from build123d import *

# Parameters (mm, degrees)
DODANIE_WYCI_GNI_CIE1_DEPTH      = 345
DODANIE_WYCI_GNI_CIE1_DEPTH_BACK = 345
SZKIC1_W                         = 200
SZKIC1_H                         = 600
SZKIC2_R                         = 6
SZKIC2_W                         = 660
SZKIC2_H                         = 300
WYTNIJ_WYCI_GNI_CIE1_DEPTH       = 500.024047517
WYTNIJ_WYCI_GNI_CIE2_DEPTH       = 760.012516366
WYTNIJ_WYCI_GNI_CIE3_DEPTH       = 760.012516366
SZKIC5_W                         = 660
SZKIC5_H                         = 130
WYTNIJ_WYCI_GNI_CIE5_DEPTH       = 469.001068375
ZAOKR_GLENIE1_R                  = 20
LUSTRO1_START                    = 330
LUSTRO1_DEPTH                    = 15
LUSTRO1_2_DEPTH                  = 15


# Read off the part's stored shape, not the designer's step: Lustro1
with BuildPart() as part:
    # Szkic1 → Dodanie-wyciągnięcie1 (new, two sides: drawn at the far end of the back side and taken through both)
    with BuildSketch(Plane(origin=(0, 0, 0), x_dir=(0, 0, -1), z_dir=(1, 0, 0)).offset(-DODANIE_WYCI_GNI_CIE1_DEPTH_BACK)):
        Rectangle(SZKIC1_W, SZKIC1_H)
    extrude(amount=DODANIE_WYCI_GNI_CIE1_DEPTH + DODANIE_WYCI_GNI_CIE1_DEPTH_BACK)

    # Szkic2 → Wytnij-wyciągnięcie1 (cut, through all)
    with BuildSketch(Plane.XY.offset(100)):
        with Locations((-150, 240)):
            Circle(SZKIC2_R)
        with Locations((-150, 60)):
            Circle(SZKIC2_R)
        with Locations((150, 60)):
            Circle(SZKIC2_R)
        with Locations((150, 240)):
            Circle(SZKIC2_R)
        with Locations((0, -150)):
            Rectangle(SZKIC2_W, SZKIC2_H)
    extrude(amount=-WYTNIJ_WYCI_GNI_CIE1_DEPTH, mode=Mode.SUBTRACT)

    # Szkic3 → Wytnij-wyciągnięcie2 (cut, through all)
    with BuildSketch(Plane.ZY.offset(345)):
        Polygon((45, -110), (100, -165), (100, 300), (45, 300), align=None)
        Polygon((30, 300), (-100, 0), (-100, 300), align=None)
    extrude(amount=-WYTNIJ_WYCI_GNI_CIE2_DEPTH, mode=Mode.SUBTRACT)

    # Szkic4 → Wytnij-wyciągnięcie3 (cut, through all)
    with BuildSketch(Plane.ZY.offset(345)):
        with BuildLine():
            Line((-20, -285), (36, -285))
            ThreePointArc((36, -285), (69.941125497, -270.941125497), (84, -237))
            Line((84, -237), (84, -207))
            ThreePointArc((84, -207), (80, -203), (76, -207))
            Line((76, -207), (76, -237))
            ThreePointArc((76, -237), (64.284271247, -265.284271247), (36, -277))
            Line((36, -277), (-20, -277))
            ThreePointArc((-20, -277), (-24, -281), (-20, -285))
        make_face()
        with BuildLine():
            Line((77.171572875, -179.828427125), (33.171572875, -135.828427125))
            ThreePointArc((33.171572875, -135.828427125), (33.171572875, -130.171572875), (38.828427125, -130.171572875))
            Line((38.828427125, -130.171572875), (82.828427125, -174.171572875))
            ThreePointArc((82.828427125, -174.171572875), (82.828427125, -179.828427125), (77.171572875, -179.828427125))
        make_face()
        with BuildLine():
            Line((8.171572875, -110.828427125), (-64.580770724, -38.076083526))
            ThreePointArc((-64.580770724, -38.076083526), (-65.447861729, -33.716922672), (-61.752343599, -31.247656401))
            Line((-61.752343599, -31.247656401), (11, -31.247656401))
            ThreePointArc((11, -31.247656401), (13.828427125, -32.419229276), (15, -35.247656401))
            Line((15, -35.247656401), (15, -108))
            ThreePointArc((15, -108), (12.530733729, -111.69551813), (8.171572875, -110.828427125))
        make_face()
        with BuildLine():
            Line((-61.752343599, -1.247656401), (11, -1.247656401))
            ThreePointArc((11, -1.247656401), (13.828427125, -0.076083526), (15, 2.752343599))
            Line((15, 2.752343599), (15, 170.642367288))
            ThreePointArc((15, 170.642367288), (11.812129914, 174.559055303), (7.329777499, 172.232797039))
            Line((7.329777499, 172.232797039), (-65.4225661, 4.342773349))
            ThreePointArc((-65.4225661, 4.342773349), (-65.096122823, 0.557089514), (-61.752343599, -1.247656401))
        make_face()
        with BuildLine():
            Line((33.95836944, -179.04163056), (-73.171572875, -71.911688245))
            ThreePointArc((-73.171572875, -71.911688245), (-77.530733729, -71.04459724), (-80, -74.74011537))
            Line((-80, -74.74011537), (-80, -141.933358006))
            ThreePointArc((-80, -141.933358006), (-79.863703305, -142.968634187), (-79.464101615, -143.933358006))
            Line((-79.464101615, -143.933358006), (-27.704526957, -233.583571092))
            ThreePointArc((-27.704526957, -233.583571092), (-24.762530111, -235.549350538), (-21.411998217, -234.411998217))
            Line((-21.411998217, -234.411998217), (33.95836944, -179.04163056))
        make_face()
        Polygon((-24, -300), (-100, -168.364138625), (-100, -300), align=None)
    extrude(amount=-WYTNIJ_WYCI_GNI_CIE3_DEPTH, mode=Mode.SUBTRACT)

    # Szkic5 → Wytnij-wyciągnięcie5 (cut, through all)
    with BuildSketch(Plane(origin=(0, 0, 0), x_dir=(1, 0, 0), z_dir=(0, 1, 0))):
        with Locations((0, 35)):
            Rectangle(SZKIC5_W, SZKIC5_H)
    extrude(amount=WYTNIJ_WYCI_GNI_CIE5_DEPTH, mode=Mode.SUBTRACT)

    # Zaokrąglenie1
    zaokr_glenie1_edges = [part.edges().sort_by_distance(p)[0] for p in [
        (-337.5, -300, -24),
        (-337.5, -168.364138625, -100),
        (-337.5, -110, 45),
        (-337.5, -165, 100),
        (-337.5, -300, 100),
        (-337.5, 0, -100),
    ]]
    fillet(zaokr_glenie1_edges, radius=ZAOKR_GLENIE1_R)

    # Lustro1 outline → Lustro1 (cut)
    with BuildSketch(Plane.YZ.offset(LUSTRO1_START)):
        with BuildLine():
            ThreePointArc((3.805124986, -98.351112506), (-0.086374196, -99.583440072), (-4.147023767, -100))
            Line((-4.147023767, -100), (0, -100))
            Line((0, -100), (3.805124986, -98.351112506))
        make_face()
        with BuildLine():
            ThreePointArc((-163.005154776, -100), (-168.181535678, -99.318516526), (-173.005154776, -97.320508076))
            Line((-173.005154776, -97.320508076), (-168.364138625, -100))
            Line((-168.364138625, -100), (-163.005154776, -100))
        make_face()
        with BuildLine():
            ThreePointArc((-290, -29.773502692), (-297.320508076, -22.452994616), (-300, -12.452994616))
            Line((-300, -12.452994616), (-300, -24))
            Line((-300, -24), (-290, -29.773502692))
        make_face()
        with BuildLine():
            ThreePointArc((-300, 80), (-294.142135624, 94.142135624), (-280, 100))
            Line((-280, 100), (-300, 100))
            Line((-300, 100), (-300, 80))
        make_face()
        with BuildLine():
            ThreePointArc((-173.284271247, 100), (-165.6306026, 98.47759065), (-159.142135624, 94.142135624))
            Line((-159.142135624, 94.142135624), (-165, 100))
            Line((-165, 100), (-173.284271247, 100))
        make_face()
    extrude(amount=LUSTRO1_DEPTH, mode=Mode.SUBTRACT)

    # Lustro1 2 outline → Lustro1 2 (add)
    with BuildSketch(Plane.YZ.offset(LUSTRO1_START)):
        with BuildLine():
            ThreePointArc((-101.715728753, 45), (-109.3693974, 46.52240935), (-115.857864376, 50.857864376))
            Line((-115.857864376, 50.857864376), (-110, 45))
            Line((-110, 45), (-101.715728753, 45))
        make_face()
    extrude(amount=LUSTRO1_2_DEPTH)


solid = part.part
Build history of the part. All positions in model axes, mm. A direction names the side the tool comes from. Give positions to 0.01 mm unless a question says otherwise; leave off trailing zeros. Loops run counter-clockwise (first coordinate to the right, second up) from the corner with the lowest first, then second, coordinate; pieces in that order, holes last. Notation, with made-up numbers: (-34, 73) - (9, 73) arc R18 ccw to (9, 79) - close; hole circle Ø10 at (-18.75, -26.5). An arc over 180 degrees is marked (long way). Write item = value, one per line. Start each with the question number.
1) Band-saw the part on B-B on x = 73. Give the cut face in (y, z).
2) Drop flat-ended pins along their axis: pin 1 Ø11 at (x, y) = (-150, 240) entering from +Z; pin 2 Ø7.5 at (x, z) = (-336.5, 15.5) entering from +Y; pin 3 Ø8 at (x, y) = (88.5, 148) entering from +Z; pin 4 Ø7.5 at (x, y) = (-338.5, -221) entering from -Z. Give the stop position or say it passes through.
3) Pull direction Y, two halves, no side cores. Call faces 1 (the flat face through (337.395, 153.976, -33.277)), 2 (the flat face through (337.395, -188.131, -53.947)), 3 (the flat face through (337, -300, 34)), 4 (the flat face through (-330, -71, 24)): +Y half, -Y half, draft (parallel to the pull), parting line (faces both ways), or undercut.
4) Probe probe 1 along Y at (x, z) = (150, 35); probe 2 along X at (y, z) = (-39, -67); probe 3 along Z at (x, y) = (-175.5, 248.5). List the from-to ranges inside material, lowest first. Write a range as from..to.
5) Tool access for faces 5 (the flat face through (-338, 86, 15)), 6 (the flat face through (337, -227, 100)): list every direction of +Z, -Z, +X, -X, +Y, -Y with a clear straight run to the whole face (end or side of a thin tool).
6) Band-saw the part on A-A on y = 96. Give the cut face in (x, z).
Final values:
q1.outline = (0, 30) - (300, 30) - (300, 45) - (0, 45) - close
q2.pin_1 = through
q2.pin_2 = 275.19
q2.pin_3 = 45
q2.pin_4 = -71.78
q3.face_1 = +Y half
q3.face_2 = undercut
q3.face_3 = -Y half
q3.face_4 = draft
q4.probe_1 = 0..54, 66..234, 246..300
q4.probe_2 = -345..-330, 330..345
q4.probe_3 = 30..45
q5.face_5 = +X, -X
q5.face_6 = +Z, +X, -X, +Y, -Y
q6.outline = (-345, -58.4) - (-330, -58.4) - (-330, -25.7) - (-345, -25.7) - close; (-345, 15) - (-330, 15) - (-330, 30) - (330, 30) - (330, 15) - (345, 15) - (345, 45) - (-345, 45) - close; (330, -58.4) - (345, -58.4) - (345, -25.7) - (330, -25.7) - close
